```python
from build123d import *

# Parameters (mm, degrees)
CROQUIS1_W              = 50.8
CROQUIS1_H              = 6.31
SALIENTE_EXTRUIR1_DEPTH = 330.7
CROQUIS3_W              = 50.8
CROQUIS3_H              = 6.31
SALIENTE_EXTRUIR2_DEPTH = 544.51
CROQUIS4_W              = 50.8
CROQUIS4_H              = 6.31


with BuildPart() as part:
    # Croquis1 → Saliente-Extruir1 (new body)
    with BuildSketch(Plane.XY):
        Rectangle(CROQUIS1_W, CROQUIS1_H)
    extrude(amount=SALIENTE_EXTRUIR1_DEPTH)

    # Croquis3 → Saliente-Extruir2 (add)
    with BuildSketch(Plane.XZ.offset(3.155)):
        with Locations((0, 3.155)):
            Rectangle(CROQUIS3_W, CROQUIS3_H)
    extrude(amount=-SALIENTE_EXTRUIR2_DEPTH)

    # Barrer1: sweep along a curve in space
    with BuildLine() as barrer1_path:
        Line((0, 541.355, 3.155), (0, 551.355, 3.155))
        Line((0, 551.355, 3.155), (0, 551.355, 44.965))
        Line((0, 551.355, 44.965), (0, 634.515, 44.965))
    # Croquis4 → Barrer1 (sweep)
    with BuildSketch(Plane(origin=(0, 541.355, 0), x_dir=(1, 0, 0), z_dir=(0, 1, 0))):
        with Locations((0, -3.155)):
            Rectangle(CROQUIS4_W, CROQUIS4_H)
    sweep(path=barrer1_path.line, transition=Transition.RIGHT)


solid = part.part
```
Source: CAD feature listing. Evaluate the final solid. Frame: model axes, mm. A direction names the side the tool comes from. Round coordinates to 2 decimals unless told otherwise and drop trailing zeros. Loops run counter-clockwise (first coordinate to the right, second up) from the corner with the lowest first, then second, coordinate; pieces in that order, holes last.
1. Ray query, L1, parallel to Y at x = 6.5, z = 13.5 (3 decimals); L2, parallel to Z at x = 18.5, y = 328; L3, parallel to Y at x = 22, z = 77.5 (3 decimals). Return the intervals inside material, ascending.
2. Mould query, pull axis Y, two halves, no side actions, for faces 4 (the flat face through (0, 595, 41.81)), 5 (the flat face through (0, 548.2, 28)), 6 (the flat face through (0, -3.155, 163)). Classes: released by +Y, released by -Y, zero draft, split by the parting line, or undercut.
3. Contact query for flat-ended pins moving along their axis: pin 1 (5 mm diameter, centred on x = 6, y = 263, fed in from +Z); pin 2 (3 mm diameter, centred on x = -4.5, y = 349.5, fed in from -Z); pin 3 (15 mm diameter, centred on x = -1.5, y = 579.5, fed in from +Z). Output: stop coordinate, or through.
4. Section query B-B on x = -13. Output: boundary loops of the cut face in (y, z) (3 decimals).
5. Section query D-D on z = 147.5. Output: boundary loops of the cut face in (x, y) (3 decimals), and give its area (3 significant figures).
6. Section query A-A on z = 27. Output: boundary loops of the cut face in (x, y) (3 decimals), and give its area (3 significant figures).
7. Section query C-C on y = 510. Output: boundary loops of the cut face in (x, z), and give its area (3 significant figures).
8. Access query for faces 1 (the flat face through (0, 592, 48.12)), 2 (the flat face through (0, 554.51, 21)), 3 (the flat face through (0, 279, 6.31)). Directions: +Z, -Z, +X, -X, +Y, -Y. A direction counts if a zero-diameter tool reaches every point of the face in a straight line with its end or side. Return the directions, or none.
Answers below:
1. L1: y = -3.155 to 3.155, 548.2 to 554.51
1. L2: z = 0 to 6.31
1. L3: y = -3.155 to 3.155
2. face 4: zero draft
2. face 5: undercut
2. face 6: released by -Y
3. pin 1: stops at z = 6.31
3. pin 2: stops at z = 0
3. pin 3: stops at z = 48.12
4. outline: (-3.155, 0) - (554.51, 0) - (554.51, 41.81) - (634.515, 41.81) - (634.515, 48.12) - (548.2, 48.12) - (548.2, 6.31) - (3.155, 6.31) - (3.155, 330.7) - (-3.155, 330.7) - close
5. outline: (-25.4, -3.155) - (25.4, -3.155) - (25.4, 3.155) - (-25.4, 3.155) - close
5. area: 321 mm2
6. outline: (-25.4, -3.155) - (25.4, -3.155) - (25.4, 3.155) - (-25.4, 3.155) - close; (-25.4, 548.2) - (25.4, 548.2) - (25.4, 554.51) - (-25.4, 554.51) - close
6. area: 641 mm2
7. outline: (-25.4, 0) - (25.4, 0) - (25.4, 6.31) - (-25.4, 6.31) - close
7. area: 321 mm2
8. face 1: +Z, +X, -X, +Y
8. face 2: -Z, +X, -X, +Y
8. face 3: +Z, +X, -X
